```python
from build123d import *

# Parameters (mm, degrees)
SKETCH_W        = 19
SKETCH_H        = 27
PAD_DEPTH       = 1.5
PAD001_DEPTH    = 0.2
SKETCH003_W     = 12.864
SKETCH003_H     = 23.74
POCKET_DEPTH    = 1
CHAMFER_SIZE    = 1
CHAMFER001_SIZE = 1
CHAMFER002_SIZE = 1
CHAMFER003_SIZE = 1


with BuildPart() as part:
    # Sketch → Pad (new body)
    with BuildSketch(Plane.XY):
        with Locations((9.5, 13.5)):
            Rectangle(SKETCH_W, SKETCH_H)
    extrude(amount=PAD_DEPTH)

    # Sketch001 (on Face5 of Pad) → Pad001 (join)
    with BuildSketch(Plane(origin=(0, 0, 0), x_dir=(1, 0, 0), z_dir=(0, 0, -1))):
        Polygon((18, -7.5), (24, -7.5), (27, -2.5), (31, -2.5), (31, -24.5), (27, -24.5), (24, -19.5), (18, -19.5), align=None)
    extrude(amount=-PAD001_DEPTH)

    # Sketch003 (on Face5 of Pad001) → Pocket (cut)
    with BuildSketch(Plane.XY.offset(1.5)):
        with Locations((7.532, 13.348)):
            Rectangle(SKETCH003_W, SKETCH003_H)
    extrude(amount=-POCKET_DEPTH, mode=Mode.SUBTRACT)

    # Chamfer
    chamfer_edges = [part.edges().sort_by_distance(p)[0] for p in [
        (19, 13.5, 1.5),
    ]]
    chamfer(chamfer_edges, length=CHAMFER_SIZE)

    # Chamfer001
    chamfer001_edges = [part.edges().sort_by_distance(p)[0] for p in [
        (18, 13.5, 1.5),
    ]]
    chamfer(chamfer001_edges, length=CHAMFER001_SIZE)

    # Chamfer002
    chamfer002_edges = [part.edges().sort_by_distance(p)[0] for p in [
        (17, 13.5, 1.5),
    ]]
    chamfer(chamfer002_edges, length=CHAMFER002_SIZE)

    # Chamfer003
    chamfer003_edges = [part.edges().sort_by_distance(p)[0] for p in [
        (16, 13.5, 1.5),
    ]]
    chamfer(chamfer003_edges, length=CHAMFER003_SIZE)


solid = part.part
```
Could you check a few things on this model? Use its own coordinates, in mm. A direction names the side the tool comes from. Give positions to 0.01 mm unless a question says otherwise; leave off trailing zeros. Order: outer loops, then holes, each group sorted by start corner. A loop starts at its lowest first (then second) coordinate and runs counter-clockwise, first axis right, second up.
Q1. For faces 5 (the flat face through (7, 25.218, 1)), 6 (the flat face through (15, 14, 0)), 7 (the flat face through (26, 13, 0.2)), which set-ups out of +Z, -Z, +X, -X, +Y, -Y let a thin tool reach every point of the face, with its end or its side?
Q2. Suppose I cut it at B-B, the plane x = 10.5. Write out the boundary of the cut face in (y, z), and give its area (3 significant figures).
Q3. I'm going to push flat-ended pins straight in: P1, Ø4, axis at x = 6.5, y = 13, coming from the +Z side; P2, Ø3.5, axis at x = 23.5, y = 12, coming from the +Z side; P3, Ø0.8, axis at y = 13, z = 1, coming from the +X side. Where does each tip first touch, or does it pass through?
Q4. Suppose I cut it at D-D, the plane y = 15.75. Write out the boundary of the cut face in (x, z).
Q5. Suppose I cut it at A-A, the plane y = 3.5. Write out the boundary of the cut face in (x, z), and give its area (3 significant figures).
Q6. Suppose I cut it at C-C, the plane y = 23.25. Write out the boundary of the cut face in (x, z).
Q7. If I drill on line 1 along Y through (x, z) = (4.5, 0.7); line 2 along X through (y, z) = (2.5, 0.4); line 3 along X through (y, z) = (6.25, 0.95), over which ranges is the centre line in solid material (lowest first)?
Q8. We'd pull the mould along X, two halves only. Please class faces 1 (the flat face through (9, 0, 1)), 2 (the flat face through (16, 13.3, 1.4)), 3 (the flat face through (13.964, 13, 1)), 4 (the flat face through (0, 13, 1)): +X half, -X half, draft (parallel to the pull), parting line (faces both ways), or undercut.
Solution:
1. face 5: +Z
1. face 6: -Z, +X, -X, +Y, -Y
1. face 7: +Z, +X, +Y, -Y
2. outline: (0, 0) - (27, 0) - (27, 1.5) - (25.22, 1.5) - (25.22, 0.5) - (1.48, 0.5) - (1.48, 1.5) - (0, 1.5) - close
2. area: 16.8 mm2
3. P1: stops at z = 0.5
3. P2: stops at z = 0.2
3. P3: stops at x = 18.9
4. outline: (0, 0) - (31, 0) - (31, 0.2) - (19, 0.2) - (19, 0.5) - (18.71, 0.79) - (17.92, 1.12) - (16.98, 1.3) - (15, 1.5) - (13.96, 1.5) - (13.96, 0.5) - (1.1, 0.5) - (1.1, 1.5) - (0, 1.5) - close
5. outline: (0, 0) - (19, 0) - (19, 0.5) - (18.71, 0.79) - (17.92, 1.12) - (16.98, 1.3) - (15, 1.5) - (13.96, 1.5) - (13.96, 0.5) - (1.1, 0.5) - (1.1, 1.5) - (0, 1.5) - close; (26.4, 0) - (31, 0) - (31, 0.2) - (26.4, 0.2) - close
5. area: 15.4 mm2
6. outline: (0, 0) - (19, 0) - (19, 0.5) - (18.71, 0.79) - (17.92, 1.12) - (16.98, 1.3) - (15, 1.5) - (13.96, 1.5) - (13.96, 0.5) - (1.1, 0.5) - (1.1, 1.5) - (0, 1.5) - close; (26.25, 0) - (31, 0) - (31, 0.2) - (26.25, 0.2) - close
7. line 1: y = 0 to 1.48, 25.22 to 27
7. line 2: x = 0 to 19
7. line 3: x = 0 to 1.1, 13.96 to 18.33
8. face 1: draft
8. face 2: +X half
8. face 3: undercut
8. face 4: -X half
